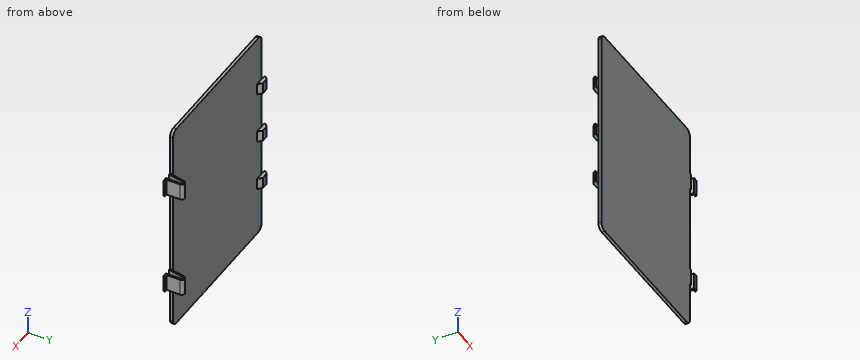
Autodesk Inventor part; units mm, degrees
ref_plane "РабПлоскость1" through (-48, 0, 40.75) normal (0, 0, 1) x (1, 0, 0)
ref_plane "РабПлоскость3" through (-55, 2, 17.5) normal (0, 0, 1) x (1, 0, 0)
ref_plane "YZ Plane" through (0, 0, 0) normal (1, 0, 0) x (0, 1, 0)
sketch "Эскиз1" plane through (0, 0, 0) normal (0, 1, 0) x (-1, 0, 0)
  line L0 (-48, -71.75) -> (48, -71.75)
  line L1 (52, -67.75) -> (52, 67.75)
  line L2 (48, 71.75) -> (-48, 71.75)
  line L3 (-52, 67.75) -> (-52, -67.75)
  line L4 (-52, -71.75) -> (52, 71.75) construction
  line L5 (52, -71.75) -> (-52, 71.75) construction
  arc A0 (52, 67.75) -> (48, 71.75) centre (48, 67.75) ccw
  arc A1 (48, -71.75) -> (52, -67.75) centre (48, -67.75) ccw
  arc A2 (-52, -67.75) -> (-48, -71.75) centre (-48, -67.75) ccw
  arc A3 (-48, 71.75) -> (-52, 67.75) centre (-48, 67.75) ccw
  line L6 (-52, 40.75) -> (-54, 40.75)
  line L7 (-54, 40.75) -> (-54, 29.75)
  line L8 (-54, 29.75) -> (-52, 29.75)
  line L9 (-52, 29.75) -> (-52, 40.75)
  line L10 (-52, 0) -> (52, 0)
  line L11 (-52, -40.75) -> (-54, -40.75)
  line L12 (-54, -40.75) -> (-54, -29.75)
  line L13 (-54, -29.75) -> (-52, -29.75)
  line L14 (-52, -29.75) -> (-52, -40.75)
  circle A4 centre (-30, -63.75) radius 2.05
  line L15 (0, -71.75) -> (0, 71.75)
  circle A5 centre (30, -63.75) radius 2.05
  circle A6 centre (-30, 63.75) radius 2.05
  circle A7 centre (30, 63.75) radius 2.05
  point P0 (0, 0)
  point P1 (-52, 29.75)
  point P2 (-52, -29.75)
  point P3 (-52, -40.75)
  dimension "d0" = 104
  dimension "d1" = 143.5
  dimension "d2" = 4
  dimension "d3" = 2
  dimension "d4" = 11
  dimension "d5" = 31
  dimension "d6" = 4.1
  dimension "d7" = 8
  dimension "d8" = 60
extrude "Выдавливание1" add sketch "Эскиз1" along normal blind 2 contours A2 L3 L10 L15 L0 | L15 L10 L1 A1 L0 | L15 L2 A0 L1 L10 | L10 L3 A3 L2 L15 | A4 | A5 | A6 | A7
ref_plane "РабПлоскость1" through (-48, 0, 40.75) normal (0, 0, 1) x (1, 0, 0)
sketch "Эскиз3" plane through (-48, 0, 40.75) normal (0, 0, 1) x (1, 0, 0)
  line L0 (100, 0) -> (102.0373, 10.3941)
  arc A0 (106, 10.0094) -> (102.0373, 10.3941) centre (104, 10.0094) ccw
  line L1 (100, 2) -> (96, 2)
  line L2 (106, 10.0094) -> (106, 1.1)
  line L3 (101.1209, 0) -> (103.1168, 10.1825)
  arc A1 (104.9, 10.0094) -> (103.1168, 10.1825) centre (104, 10.0094) ccw
  line L4 (104.9, 10.0094) -> (104.9, 0)
  line L5 (100, 0) -> (96, 0)
  line L6 (100, 0) -> (101.1209, 0)
  line L7 (104.9, 0) -> (109, 0)
  line L8 (104.9, 0) -> (107.9, 0)
  line L9 (107.9, 0) -> (107.9, 1.1)
  line L10 (107.9, 1.1) -> (106, 1.1)
  line L11 (104.9, 1.1) -> (104.9, 0)
  line L12 (100, 2) -> (100.392, 2)
  line L13 (100, 2) -> (100, 0)
  point P0 (48, 0)
  point P1 (104.1933, 12)
  dimension "d19" = 10
  dimension "d20" = 2
  dimension "d21" = 6
  dimension "d22" = 1.1
  dimension "d23" = 1.1
  dimension "d24" = 1.1
  dimension "d25" = 3
extrude "Выдавливание2" add sketch "Эскиз3" against normal blind 11
mirror "Зеркальное отражение1" about plane through (0, 0, 0) normal (0, 0, 1) of "Выдавливание2"
sketch "Эскиз4" plane through (0, 2, 0) normal (0, 1, 0) x (1, 0, 0)
  line L0 (-46.5, -31.25) -> (-55, -31.25)
  line L1 (-55, -31.25) -> (-55, -38.75)
  line L2 (-55, -38.75) -> (-46.5, -38.75)
  line L3 (-46.5, -38.75) -> (-46.5, -31.25)
  line L4 (-52, 67.75) -> (-52, -67.75)
  line L5 (-48, -71.75) -> (48, -71.75)
  point P0 (0, 0)
  dimension "d28" = 7.5
  dimension "d29" = 3
  dimension "d30" = 33
  dimension "d31" = 5.5
extrude "Выдавливание3" add sketch "Эскиз4" along normal blind 2.5
mirror "Зеркальное отражение2" about plane through (0, 0, 0) normal (0, 0, 1) of "Выдавливание3"
ref_plane "РабПлоскость3" through (-55, 2, 17.5) normal (0, 0, 1) x (1, 0, 0)
ref_plane "РабПлоскость2" through (-55, 2, 35) normal (0, 0, 1) x (1, 0, 0)
mirror "Зеркальное отражение3" about plane through (-55, 2, 17.5) normal (0, 0, 1) of "Выдавливание3"
chamfer "Фаска1" distance 1.5 angle 45 3 edges at (-55, 4.5, 35) (-55, 4.5, 0) (-55, 4.5, -35)
chamfer "Фаска2" distance 2.5 angle 45 3 edges at (-46.5, 4.5, 35) (-46.5, 4.5, -35) (-46.5, 4.5, 0)
properties part number "Toolbox cover"
Work out the finished part from the listing and answer in its coordinate system (mm). Round coordinates to 2 decimals unless told otherwise and drop trailing zeros. Write each loop counter-clockwise with the first axis right and the second up, starting at its lowest first coordinate (ties: lowest second). Pieces come first, ordered by that corner, then holes. Notation, with made-up numbers: (-18, 19) - (9, 19) arc R14 cw to (9, 40) - close; hole circle Ø11 at (81.25, -17). An arc over 180 degrees is marked (long way). Answer in a Markdown table with one row per item. Add a question column.
1. Find the intervals of material crossed by line 1 along Y through (x, z) = (-20.5, -41); line 2 along X through (y, z) = (4, -39); line 3 along X through (y, z) = (1, 55.5), in increasing order. Write a range as from..to.
2. A cutting plane is placed at A-A, the plane y = 6. Determine the outline of the cut face in (x, z).
3. A cutting plane is placed at C-C, the plane z = 25. Determine the outline of the cut face in (x, y), and give its area (3 significant figures).
4. A cutting plane is placed at B-B, the plane x = 16. Determine the outline of the cut face in (y, z).
5. Given pin 1 (3.5 mm diameter, centred on x = -54, z = -36, fed in from -Y); pin 2 (3 mm diameter, centred on x = 34.5, z = -24, fed in from +Y); pin 3 (1.2 mm diameter, centred on x = -53, y = 2.5, fed in from +Z); pin 4 (3.5 mm diameter, centred on x = -53, z = 34, fed in from -Y), each flat-ended and moving along its own axis, determine where each tip first touches the part or whether it passes through.
Worked out:
| question | item | result |
|---|---|---|
| 1 | line 1 | 0..2 |
| 1 | line 2 | 52.78..53.9, 56.9..58 |
| 1 | line 3 | -52..52 |
| 2 | outline | (53.18, -40.75) - (54.3, -40.75) - (54.3, -29.75) - (53.18, -29.75) - close; (53.18, 29.75) - (54.3, 29.75) - (54.3, 40.75) - (53.18, 40.75) - close; (56.9, -40.75) - (58, -40.75) - (58, -29.75) - (56.9, -29.75) - close; (56.9, 29.75) - (58, 29.75) - (58, 40.75) - (56.9, 40.75) - close |
| 3 | outline | (-52, 0) - (52, 0) - (52, 2) - (-52, 2) - close |
| 3 | area | 208 mm^2 |
| 4 | outline | (0, -71.75) - (2, -71.75) - (2, 71.75) - (0, 71.75) - close |
| 5 | pin 1 | y = 2 |
| 5 | pin 2 | y = 2 |
| 5 | pin 3 | z = 38.75 |
| 5 | pin 4 | y = 0 |
